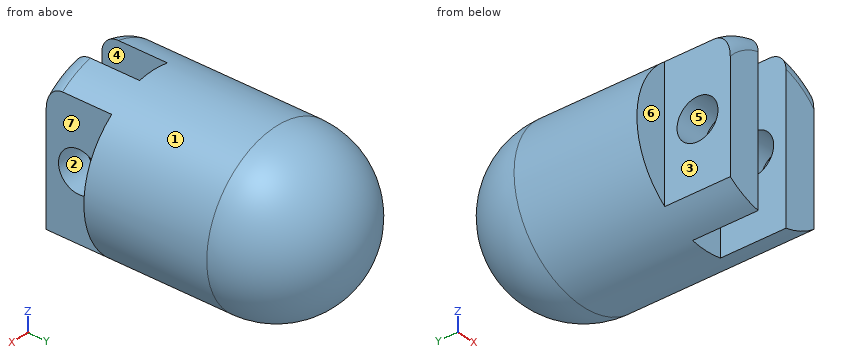
```python
from build123d import *

# Parameters (mm, degrees)
CUT_EXTRUDE1_DEPTH = 10.16
SKETCH3_R          = 3.175
CUT_EXTRUDE2_DEPTH = 49.276707634
FILLET1_R          = 2.54


with BuildPart() as part:
    # Sketch1 → Revolve1 (revolve)
    with BuildSketch(Plane.XY):
        with BuildLine():
            Line((0, 0), (0, 5.602635041))
            Line((0, 5.602635041), (-2.54, 5.602635041))
            Line((-2.54, 5.602635041), (-2.54, 22.86))
            ThreePointArc((-2.54, 22.86), (-6.715756159, 30.503336463), (0, 36.049159305))
            Line((0, 36.049159305), (0, 41.91))
            ThreePointArc((0, 41.91), (-8.980256121, 38.190256121), (-12.7, 29.21))
            Line((-12.7, 29.21), (-12.7, 0))
            Line((-12.7, 0), (0, 0))
        make_face()
    revolve(axis=Axis((0, 0, 0), (0, 1, 0)))

    # Sketch2 → Cut-Extrude1 (cut)
    with BuildSketch(Plane.XZ):
        with BuildLine():
            Line((-2.54, 12.443407893), (-2.54, -12.443407893))
            ThreePointArc((-2.54, -12.443407893), (0, -12.7), (2.54, -12.443407893))
            Line((2.54, -12.443407893), (2.54, 12.443407893))
            ThreePointArc((2.54, 12.443407893), (0, 12.7), (-2.54, 12.443407893))
        make_face()
        with BuildLine():
            Line((-7.62, 10.16), (-7.62, -10.16))
            ThreePointArc((-7.62, -10.16), (-12.7, 0), (-7.62, 10.16))
        make_face()
        with BuildLine():
            Line((7.62, 10.16), (7.62, -10.16))
            ThreePointArc((7.62, -10.16), (12.7, 0), (7.62, 10.16))
        make_face()
    extrude(amount=-CUT_EXTRUDE1_DEPTH, mode=Mode.SUBTRACT)

    # Sketch3 → Cut-Extrude2 (cut, through all)
    with BuildSketch(Plane.ZY.offset(7.62)):
        with Locations((0, 5.08)):
            Circle(SKETCH3_R)
    extrude(amount=-CUT_EXTRUDE2_DEPTH, mode=Mode.SUBTRACT)

    # Fillet1
    fillet1_edges = [part.edges().sort_by_distance(p)[0] for p in [
        (5.206715654, 0, 11.583613948),
        (-5.206715654, 0, 11.583613948),
    ]]
    fillet(fillet1_edges, radius=FILLET1_R)


solid = part.part
```
Can you work these out from the model? Positions are in its coordinate system, mm. Face numbers are marked on the shaded views. A direction names the side the tool comes from. Round coordinates to 2 decimals unless told otherwise and drop trailing zeros. Loops run counter-clockwise (first coordinate to the right, second up) from the corner with the lowest first, then second, coordinate; pieces in that order, holes last. Notation, with made-up numbers: M 33.25,67 L 83.25,67 A22 cw 83.25,81 Z; hole C 79.25,50 d10. An arc over 180 degrees is marked long. Write item = value, one per line. Start each with the question number.
(1) Suppose I cut it at D-D on z = -8. Write out the boundary of the cut face in (x, y).
(2) I need wall thicknesses on line 1 along Y through (x, z) = (-6.25, 0.75); line 2 along Z through (x, y) = (0, 29); line 3 along X through (y, z) = (8, 3.5). Which ranges of each line are inside material? Lowest first, please.
(3) Which directions (+Z, -Z, +X, -X, +Y, -Y) give clear straight access to the entire face, cutting with the end or side of a thin tool? Please do the marked faces 4, 5, 6 and 7.
(4) Suppose I cut it at C-C on x = 0. Write out the boundary of the cut face in (y, z).
(5) Suppose I cut it at B-B on z = -1.25. Write out the boundary of the cut face in (x, y).
(6) Suppose I cut it at A-A on y = 5.08. Write out the boundary of the cut face in (x, z) (3 decimals), plus the area to 3 significant figures.
(7) I'm going to push flat-ended pins straight in: P1, Ø4, axis at y = 5.08, z = 0, coming from the -X side; P2, Ø3, axis at y = 4.5, z = 3.5, coming from the +X side; P3, Ø1, axis at x = 2, z = -9.5, coming from the -Y side; P4, Ø1.5, axis at x = 8, y = 20.5, coming from the -Z side. Where does each tip first touch, or does it pass through?
(8) If we mould it in two halves opening along Z, with no side actions, what happens to the marked faces 1, 2 and 3? For each: released by +Z, released by -Z, zero draft, split by the parting line, or undercut.
Answer block:
q1.outline = M -9.86,10.16 L -7.62,10.16 L -7.62,0 L -2.54,0 L -2.54,10.16 L 2.54,10.16 L 2.54,0 L 7.62,0 L 7.62,10.16 L 9.86,10.16 L 9.86,29.21 A9.86 ccw -9.86,29.21 Z
q2.line_1 = 0 to 1.99, 8.17 to 26.54, 31.88 to 40.24
q2.line_2 = -12.7 to -6.84, 6.84 to 12.7
q2.line_3 = -7.62 to -2.54, 2.54 to 7.62
q3.face_4 = +Z, -Z, -Y
q3.face_5 = +X, -X
q3.face_6 = +Z, -Z, -X, -Y
q3.face_7 = +Z, -Z, +X, -Y
q4.outline = M 10.16,-12.7 L 29.21,-12.7 A12.7 ccw 29.21,12.7 L 10.16,12.7 L 10.16,2.54 L 22.86,2.54 A6.84 cw long 22.86,-2.54 L 10.16,-2.54 Z
q5.outline = M -12.64,10.16 L -7.62,10.16 L -7.62,8 L -2.54,8 L -2.54,10.16 L -2.21,10.16 L -2.21,22.86 A6.72 cw long 2.21,22.86 L 2.21,10.16 L 2.54,10.16 L 2.54,8 L 7.62,8 L 7.62,10.16 L 12.64,10.16 L 12.64,29.21 A12.64 ccw -12.64,29.21 Z; M -7.62,0 L -2.54,0 L -2.54,2.16 L -7.62,2.16 Z; M 2.54,0 L 7.62,0 L 7.62,2.16 L 2.54,2.16 Z
q6.outline = M -7.62,-10.16 A12.7 ccw -2.54,-12.443 L -2.54,-3.175 L -7.62,-3.175 Z; M -7.62,3.175 L -2.54,3.175 L -2.54,12.443 A12.7 ccw -7.62,10.16 Z; M 2.54,-12.443 A12.7 ccw 7.62,-10.16 L 7.62,-3.175 L 2.54,-3.175 Z; M 2.54,3.175 L 7.62,3.175 L 7.62,10.16 A12.7 ccw 2.54,12.443 Z
q6.area = 170 mm²
q7.P1 = through
q7.P2 = 7.62
q7.P3 = 10.16
q7.P4 = -10.43
q8.face_1 = split by the parting line
q8.face_2 = undercut
q8.face_3 = zero draft
